Source: three-view drawing plus pictorial views. Frame: mm from the lowest corner of the part. A direction names the side the tool comes from. Give positions to 0.01 mm unless a question says otherwise; leave off trailing zeros. Loops run counter-clockwise (first coordinate to the right, second up) from the corner with the lowest first, then second, coordinate; pieces in that order, holes last. Notation, with made-up numbers: (2.5, 40.25) - (55.5, 40.25) arc R19 cw to (55.5, 44.25) - close; hole circle Ø6 at (68.5, 71.25). An arc over 180 degrees is marked (long way). Write each question's results on one line, items separated by ' | '. Start each with the question number.
(1) Cut plane C-C on z = 916.5. Return the cut outline in (x, y).
(2) Material intervals for line 1 along Z through (x, y) = (577.5, 384); line 2 along Z through (x, y) = (508, 650); line 3 along X through (y, z) = (878, 1097), sorted ascending. Write a range as [from, to].
(3) Cut plane D-D on y = 1209. Return the cut outline in (x, z), then the cut area to 3 significant figures.
(4) Contact query for flat-ended pins moving along their axis: pin 1 (1.5 mm diameter, centred on x = 254.5, y = 1054, fed in from +Z); pin 2 (3 mm diameter, centred on y = 857, z = 174.5, fed in from -X); pin 3 (1.5 mm diameter, centred on x = 890, z = 346.5, fed in from +Y). Output: stop coordinate, or through.
(5) Reachability of the marked faces 1 and 2 from +Z, -Z, +X, -X, +Y, -Y: full face, straight path, thin tool, end or side. Return the list, or none.
(6) Cut plane A-A on y = 762. Return the cut outline in (x, z).
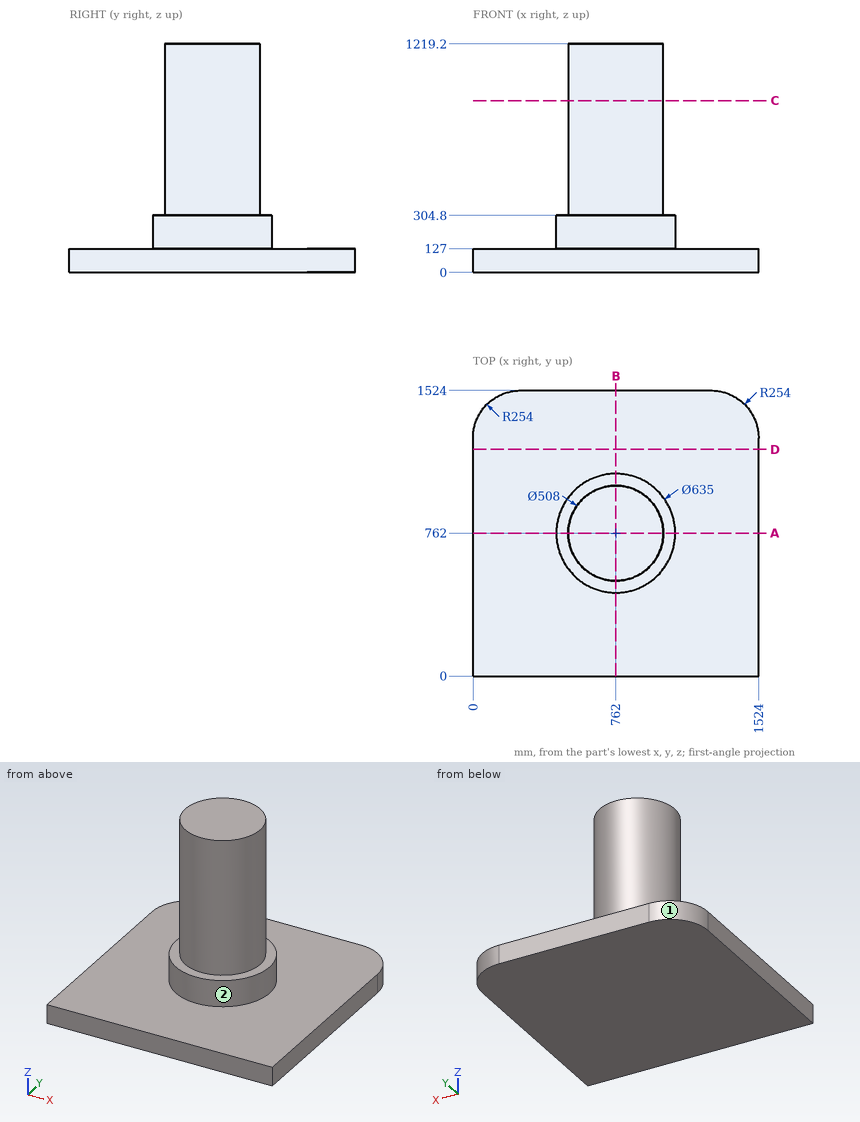
Ans:
1) outline: circle Ø508 at (762, 762)
2) line 1: [0, 127] | line 2: [0, 304.8] | line 3: [536.04, 987.96]
3) outline: (0, 0) - (1524, 0) - (1524, 127) - (0, 127) - close | area: 194,000 mm^2
4) pin 1: z = 127 | pin 2: x = 458.58 | pin 3: y = 981.83
5) face 1: +Z, -Z, -X, +Y | face 2: +Z
6) outline: (0, 0) - (1524, 0) - (1524, 127) - (1079.5, 127) - (1079.5, 304.8) - (1016, 304.8) - (1016, 1219.2) - (508, 1219.2) - (508, 304.8) - (444.5, 304.8) - (444.5, 127) - (0, 127) - close
